The model under review builds one solid part; all positions refer to its coordinate system, in mm. A direction names the side the tool comes from. Round coordinates to 2 decimals unless told otherwise and drop trailing zeros. Loops run counter-clockwise (first coordinate to the right, second up) from the corner with the lowest first, then second, coordinate; pieces in that order, holes last. Notation, with made-up numbers: (21.5, 49.5) -> (67.5, 49.5) arc R16 ccw to (67.5, 53.5) -> close; hole circle Ø8 at (88.5, -13.75). An arc over 180 degrees is marked (long way). Return JSON: item names as keys, results as strings. Group by question number.
Solid Edge part; units mm, degrees
sketch "Sketch1" plane through (0, 0, 0) normal (0, -1, 0) x (1, 0, 0)
  line L0 (73, 0) -> (0, 0)
  line L1 (0, 0) -> (0, -70)
  line L2 (0, -70) -> (73, -70)
  line L3 (73, -70) -> (73, 0)
extrude "Protrusion1" add sketch "Sketch1" against normal blind 112
sketch "Sketch2" plane through (36.5, 0, -35) normal (0, -1, 0) x (1, 0, 0)
  line L0 (-26.5, 35) -> (36.5, 35)
  line L1 (36.5, 35) -> (36.5, -16)
  line L2 (24.5, -16) -> (36.5, -16)
  arc A0 (-26.5, 35) -> (24.5, -16) centre (24.5, 35) ccw
extrude "ExtrudedCutout_1" cut sketch "Sketch2" against normal blind 26
sketch "Sketch3" plane through (41.5, 26, -25.5) normal (0, -1, 0) x (1, 0, 0)
  line L0 (31.5, 25.5) -> (-31.5, 25.5)
  line L1 (31.5, 13.5) -> (-31.5, 25.5)
  line L2 (31.5, 25.5) -> (31.5, 13.5)
extrude "ExtrudedCutout_2" cut sketch "Sketch3" against normal blind 16
sketch "Sketch4" plane through (36.5, 112, -35) normal (0, 1, 0) x (-1, 0, 0)
  line L0 (-36.5, 35) -> (-36.5, -23)
  line L1 (36.5, 35) -> (-36.5, -23)
  line L2 (36.5, 35) -> (-36.5, 35)
extrude "ExtrudedCutout_3" cut sketch "Sketch4" against normal blind 70
sketch "Sketch5" plane through (36.5, 112, -35) normal (0, 1, 0) x (-1, 0, 0)
  line L0 (13.8448, 17) -> (36.5, 35)
  line L1 (36.5, 35) -> (36.5, 17)
  line L2 (36.5, 17) -> (13.8448, 17)
extrude "ExtrudedCutout_4" cut sketch "Sketch5" against normal blind 22
sketch "Sketch6" plane through (36.5, 56, -70) normal (0, 0, -1) x (0, -1, 0)
  line L0 (-25, -21.6238) -> (-44, -21.6238)
  line L1 (-44, -21.6238) -> (-44, -9.0965)
  line L2 (-44, -9.0965) -> (-25, -9.0965)
  line L3 (-25, -9.0965) -> (-25, -21.6238)
extrude "ExtrudedCutout_6" cut sketch "Sketch6" against normal blind 64.3754
1. Tool access review of faces 1 (the face through (41.941, 33.888, -6.084)), 2 (the face through (53, 42, -23)), 3 (the face through (24.54, 12.82, -35.66)), 4 (the face through (6, 90, -13)), 5 (the face through (52, 100, -57)): name each direction out of +Z, -Z, +X, -X, +Y, -Y from which nothing blocks a thin tool from reaching the whole face with its end or side.
2. Wall thickness on line 1 (Y direction, x = 66.5, z = -27); line 2 (Z direction, x = 21.5, y = 97); line 3 (Z direction, x = 59.5, y = 15): over which ranges is each line inside the solid? List them lowest first.
3. We need section D-D, the plane y = 83.5. Write out the cut boundary in (x, z), then the cut area to 3 significant figures.
4. For P1, Ø1, axis at x = 32, y = 75.5, coming from the +Z side; P2, Ø6, axis at x = 43.5, y = 66, coming from the +Z side; P3, Ø6, axis at x = 14, z = -11.5, coming from the +Y side; P4, Ø15, axis at y = 93, z = -52.5, coming from the -X side, all flat-tipped, find the tip position at first contact; note any pin that passes through.
5. We need section C-C, the plane x = 52. Write out the cut boundary in (y, z).
6. We need section A-A, the plane y = 96.5. Write out the cut boundary in (x, z), then the cut area to 3 significant figures.
7. We need section B-B, the plane z = -38.5. Write out the cut boundary in (x, y), then the cut area to 3 significant figures.
8. Draft analysis for pull direction Y (two halves, no side actions). For faces 6 (the face through (45.596, 91, -53)), 7 (the face through (36, 55, -70)), 8 (the face through (29, 0, -50)), state which applies: pulls with the +Y half, pulls with the -Y half, needs draft (parallel to the pull), parting line crosses it, or undercut.
Check sheet entries:
{
 "1": {"face 1": "+Z, +X, +Y, -Y", "face 2": "+Z, +X, +Y", "face 3": "+Z, +X, -Y", "face 4": "+Z, +X, -X, +Y", "face 5": "+Z, -Z"},
 "2": {"line 1": "y = 26 to 42", "line 2": "z = -70 to -18", "line 3": "z = -70 to -50.98"},
 "3": {"outline": "(0, -70) -> (45.6, -70) -> (45.6, -36.23) -> (0, 0) -> close; (58.12, -70) -> (73, -70) -> (73, -58) -> (58.12, -46.18) -> close", "area": "2,630 mm²"},
 "4": {"P1": "stops at z = -25.03", "P2": "stops at z = -32.18", "P3": "stops at y = 90", "P4": "stops at x = 0"},
 "5": {"outline": "(0, -70) -> (81, -70) -> (81, -41.32) -> (42, -41.32) -> (42, -8) -> (26, -8) -> (26, -50.2) -> (0, -50.2) -> close; (100, -70) -> (112, -70) -> (112, -41.32) -> (100, -41.32) -> close"},
 "6": {"outline": "(0, -70) -> (45.6, -70) -> (45.6, -36.23) -> (22.66, -18) -> (0, -18) -> close; (58.12, -70) -> (73, -70) -> (73, -58) -> (58.12, -46.18) -> close", "area": "2,430 mm²"},
 "7": {"outline": "(0, 0) -> (27.55, 0) -> (27.55, 26) -> (73, 26) -> (73, 42) -> (48.46, 42) -> (48.46, 81) -> (45.6, 81) -> (45.6, 100) -> (48.46, 100) -> (48.46, 112) -> (0, 112) -> close", "area": "5,220 mm²"},
 "8": {"face 6": "undercut", "face 7": "needs draft", "face 8": "pulls with the -Y half"}
}
